Build history of the part. All positions in model axes, mm. A direction names the side the tool comes from. Coordinates: 2 decimals unless noted, no trailing zeros. Write each loop counter-clockwise with the first axis right and the second up, starting at its lowest first coordinate (ties: lowest second). Pieces come first, ordered by that corner, then holes.
from build123d import *

# Parameters (mm, degrees)
F0_R     = 2.413
F0_R_2   = 7.9375
F1_DEPTH = 5.842


with BuildPart() as f1:
    # F0 (on Front) → F1 (new body)
    with BuildSketch(Plane.XZ):
        with BuildLine():
            Line((-19.05, 0), (-19.05, -203.2))
            ThreePointArc((-19.05, -203.2), (0, -222.25), (19.05, -203.2))
            Line((19.05, -203.2), (19.05, 0))
            ThreePointArc((19.05, 0), (0, 19.05), (-19.05, 0))
        make_face()
        with Locations((-10.795, -190.5)):
            Circle(F0_R, mode=Mode.SUBTRACT)
        with Locations((0, -203.2)):
            Circle(F0_R_2, mode=Mode.SUBTRACT)
        with Locations((10.795, -190.5)):
            Circle(F0_R, mode=Mode.SUBTRACT)
        with BuildLine():
            ThreePointArc((7.9375, -177.8), (0, -185.7375), (-7.9375, -177.8))
            Line((-7.9375, -177.8), (-7.9375, -6.35))
            ThreePointArc((-7.9375, -6.35), (0, 1.5875), (7.9375, -6.35))
            Line((7.9375, -6.35), (7.9375, -177.8))
        make_face(mode=Mode.SUBTRACT)
        with Locations((0, 12.7)):
            Circle(F0_R, mode=Mode.SUBTRACT)
    extrude(amount=F1_DEPTH)


solid = f1.part
(1) Slice it at B-B, the plane x = 0. List the corners of the cut face in (y, z), and give its area (3 significant figures).
(2) 3-axis set-ups, long thin cutter, end or side, ignore diameter. For faces 5 (the flat face through (-7.938, -3, -93)), 6 (the flat face through (-19.05, -3, -100)): which of +Z, -Z, +X, -X, +Y, -Y reach the whole face in a straight line?
(3) Probe L1, parallel to Z at x = 0, y = -3.35; L2, parallel to X at y = -4.55, z = -190.5; L3, parallel to X at y = -3.15, z = -125. List the from-to ranges inside material, lowest first.
(4) Slice it at D-D, the plane z = -190.5. List the corners of the cut face in (x, y), and give its area (3 significant figures).
(5) Two-plate mould, pull along Z, no slides. Class faces 1 (the cylindrical face through (-0.419, -2.88, -222.245)), 2 (the cylindrical face through (0.419, -2.88, 19.045)), 3 (the flat face through (8.2, -5.842, -99.9)), 4 (the flat face through (7.938, -3, -91)): pulls with the +Z half, pulls with the -Z half, needs draft (parallel to the pull), parting line crosses it, or undercut.
(6) Slice it at C-C, the plane y = -2.4. Give the number of separate pieces and of enclosed holes in the cut face, and give its area (3 significant figures).
(7) Slice it at A-A, the plane z = -50.5. List the corners of the cut face in (x, y).
(8) Flat gauge pins, fed straight in: P1, Ø2, axis at x = -3.5, y = -0.5, coming from the +Z side; P2, Ø3, axis at x = -10.795, z = -190.5, coming from the +Y side. Where does each tip first touch, or does it go through?
Results:
1. outline: (-5.84, -222.25) - (0, -222.25) - (0, -211.14) - (-5.84, -211.14) - close; (-5.84, -195.26) - (0, -195.26) - (0, -185.74) - (-5.84, -185.74) - close; (-5.84, 1.59) - (0, 1.59) - (0, 10.29) - (-5.84, 10.29) - close; (-5.84, 15.11) - (0, 15.11) - (0, 19.05) - (-5.84, 19.05) - close
1. area: 194 mm2
2. face 5: +Y, -Y
2. face 6: +Z, -Z, -X, +Y, -Y
3. L1: z = -222.25 to -211.14, -195.26 to -185.74, 1.59 to 10.29, 15.11 to 19.05
3. L2: x = -19.05 to -13.21, -8.38 to 8.38, 13.21 to 19.05
3. L3: x = -19.05 to -7.94, 7.94 to 19.05
4. outline: (-19.05, -5.84) - (-13.21, -5.84) - (-13.21, 0) - (-19.05, 0) - close; (-8.38, -5.84) - (8.38, -5.84) - (8.38, 0) - (-8.38, 0) - close; (13.21, -5.84) - (19.05, -5.84) - (19.05, 0) - (13.21, 0) - close
4. area: 166 mm2
5. face 1: pulls with the -Z half
5. face 2: pulls with the +Z half
5. face 3: needs draft
5. face 4: undercut
6. separate pieces: 1
6. enclosed holes: 5
6. area: 5,710 mm2
7. outline: (-19.05, -5.84) - (-7.94, -5.84) - (-7.94, 0) - (-19.05, 0) - close; (7.94, -5.84) - (19.05, -5.84) - (19.05, 0) - (7.94, 0) - close
8. P1: stops at z = 18.89
8. P2: passes through
